Work out the finished part from the listing and answer in its coordinate system (mm). A direction names the side the tool comes from. Give positions to 0.01 mm unless a question says otherwise; leave off trailing zeros. Loops run counter-clockwise (first coordinate to the right, second up) from the corner with the lowest first, then second, coordinate; pieces in that order, holes last. Notation, with made-up numbers: M 36,67.25 L 74,67.25 A14 cw 74,81.25 Z; hole C 63.5,50 d9. An arc over 180 degrees is marked long. Write item = value, one per line. Start each with the question number.
1. Section D-D on z = 12 is taken. Determine the outline of the cut face in (x, y).
2. For faces 1 (the face through (-63, 12, 0)), 2 (the face through (1, 2, 19)), 3 (the face through (55, 3, -15)), determine the directions among +Z, -Z, +X, -X, +Y, -Y from which every point of the face is accessible in a straight line to the end or side of a thin tool.
3. Flat-ended cylindrical pins translate along their axes: pin 1 Ø4 at (x, y) = (50, 2.5) entering from -Z; pin 2 Ø1 at (y, z) = (9.5, -1) entering from -X. Find the tip coordinate at first contact, or state that the pin passes through.
4. Consider L1, parallel to Y at x = -45, z = 0.5; L2, parallel to X at y = 3.5, z = -5.5; L3, parallel to Y at x = 41.5, z = 13. Determine where each line is inside the solid, lowest interval first. Write a range as [from, to].
5. Section B-B on z = 0 is taken. Determine the outline of the cut face in (x, y).
6. Section A-A on x = 6 is taken. Determine the outline of the cut face in (y, z), plus the area to 3 significant figures.
7. The mould has two halves that part along Y. Classify faces 4 (the face through (1, 1, -18)), 5 (the face through (55, 1, 0)), 6 (the face through (-1, 10, -20)): released by +Y, released by -Y, zero draft, split by the parting line, or undercut.
```python
from build123d import *

# Parameters (mm, degrees)
SKETCH1_W           = 150
SKETCH1_H           = 40
BOSS_EXTRUDE1_DEPTH = 20
CUT_EXTRUDE1_START  = -1
SKETCH2_W           = 30
SKETCH2_H           = 30
CUT_EXTRUDE1_DEPTH  = 5
SKETCH7_R           = 2
CUT_EXTRUDE3_DEPTH  = 140
FILLET1_R           = 5
CUT_EXTRUDE5_START  = -25
SKETCH9_R           = 9
CUT_EXTRUDE5_DEPTH  = 50
SKETCH8_R           = 2
CUT_EXTRUDE4_DEPTH  = 62


with BuildPart() as part:
    # Sketch1 → Boss-Extrude1 (new body)
    with BuildSketch(Plane(origin=(0, 0, 0), x_dir=(1, 0, 0), z_dir=(0, 1, 0))):
        Rectangle(SKETCH1_W, SKETCH1_H)
    extrude(amount=BOSS_EXTRUDE1_DEPTH)

    # Sketch2 → Cut-Extrude1 (cut)
    with BuildSketch(Plane.XZ.offset(CUT_EXTRUDE1_START)):
        with Locations((55, 0)):
            Rectangle(SKETCH2_W, SKETCH2_H)
    extrude(amount=-CUT_EXTRUDE1_DEPTH, mode=Mode.SUBTRACT)

    # Sketch7 → Cut-Extrude3 (cut)
    with BuildSketch(Plane.ZY.offset(75)):
        with Locations((12, 3.5)):
            Circle(SKETCH7_R)
    extrude(amount=-CUT_EXTRUDE3_DEPTH, mode=Mode.SUBTRACT)

    # Fillet1
    fillet1_edges = [part.edges().sort_by_distance(p)[0] for p in [
        (0, 20, -20),
        (0, 0, -20),
        (0, 0, 20),
        (0, 20, 20),
    ]]
    fillet(fillet1_edges, radius=FILLET1_R)

    # Sketch9 → Cut-Extrude5 (cut)
    with BuildSketch(Plane.ZY.offset(75).offset(CUT_EXTRUDE5_START)):
        with Locations((0, 10)):
            Circle(SKETCH9_R)
    extrude(amount=-CUT_EXTRUDE5_DEPTH, mode=Mode.SUBTRACT)

    # Sketch8 → Cut-Extrude4 (cut)
    with BuildSketch(Plane.ZY.offset(75)):
        with Locations((0, 10)):
            Circle(SKETCH8_R)
    extrude(amount=-CUT_EXTRUDE4_DEPTH, mode=Mode.SUBTRACT)


solid = part.part
```
Verdict:
q1.outline = M -75,0 L 75,0 L 75,20 L -75,20 L -75,5.5 L 40,5.5 L 40,6 L 70,6 L 70,1 L 40,1 L 40,1.5 L -75,1.5 Z
q2.face_1 = -X
q2.face_2 = +Z, +X, -X, -Y
q2.face_3 = none
q3.pin_1 = -19.97
q3.pin_2 = 0
q4.L1 = [0, 1.01], [18.99, 20]
q4.L2 = [-75, -50], [0, 40], [70, 75]
q4.L3 = [0, 1], [6, 20]
q5.outline = M -75,0 L 75,0 L 75,20 L -75,20 L -75,12 L -50,12 L -50,19 L 0,19 L 0,1 L -50,1 L -50,8 L -75,8 Z; hole M 40,1 L 70,1 L 70,6 L 40,6 Z
q6.outline = M 0,-15 A5 ccw 5,-20 L 15,-20 A5 ccw 20,-15 L 20,15 A5 ccw 15,20 L 5,20 A5 ccw 0,15 Z; hole C 3.5,12 d4
q6.area = 766 mm2
q7.face_4 = released by -Y
q7.face_5 = undercut
q7.face_6 = zero draft
